from build123d import *

# Parameters (mm, degrees)
F1_DEPTH = 25
F2_R     = 8
F3_DEPTH = 25
F4_SIZE  = 5
F5_R     = 1.75
F6_DEPTH = 25


with BuildPart() as f1:
    # F0 (on Right) → F1 (new body)
    with BuildSketch(Plane.YZ):
        with BuildLine():
            Line((2, 47), (0, 47))
            Line((0, 47), (0, 5))
            ThreePointArc((0, 5), (1.464466, 1.464466), (5, 0))
            Line((5, 0), (52, 0))
            Line((52, 0), (52, 2))
            Line((52, 2), (5, 2))
            ThreePointArc((5, 2), (2.87868, 2.87868), (2, 5))
            Line((2, 5), (2, 47))
        make_face()
    extrude(amount=F1_DEPTH)

    # F2 (on face) → F3 (cut)
    with BuildSketch(Plane(origin=(0, 2, 0), x_dir=(-1, 0, 0), z_dir=(0, 1, 0))):
        with Locations((-12.5, 35)):
            Circle(F2_R)
    extrude(amount=-F3_DEPTH, mode=Mode.SUBTRACT)

    # F4
    f4_edges = [f1.edges().sort_by_distance(p)[0] for p in [
        (0, 1, 47),
        (25, 1, 47),
    ]]
    chamfer(f4_edges, length=F4_SIZE)

    # F5 (on face) → F6 (cut)
    with BuildSketch(Plane.XY.offset(2)):
        with Locations((12.5, 43)):
            Circle(F5_R)
        with Locations((12.5, 28)):
            Circle(F5_R)
    extrude(amount=-F6_DEPTH, mode=Mode.SUBTRACT)


solid = f1.part
CAD build for the part. Positions are in the model's coordinates, mm. A direction names the side the tool comes from. Round coordinates to 2 decimals unless told otherwise and drop trailing zeros. Write each loop counter-clockwise with the first axis right and the second up, starting at its lowest first coordinate (ties: lowest second). Pieces come first, ordered by that corner, then holes. Notation, with made-up numbers: M -17.75,74 L 20.25,74 A35 ccw 20.25,108 Z; hole C -18,8 d8. An arc over 180 degrees is marked long. Use a Markdown table: item, result. Add a question column.
1. Flat gauge pins, fed straight in: P1, Ø5, axis at x = 21.5, y = 26.5, coming from the +Z side; P2, Ø12.5, axis at x = 15.5, z = 24.5, coming from the +Y side. Where does each tip first touch, or does it go through?
2. Slice it at C-C on z = 36. Give the cut face in (x, y).
3. Drill centre lines: probe 1 along Y at (x, z) = (12.5, 1.35); probe 2 along Y at (x, z) = (12.5, 1.5); probe 3 along Z at (x, y) = (8.5, 47). Where is each one in solid material? Low to high.
4. Slice it at A-A on y = 43. Give the cut face in (x, z).
5. Slice it at B-B on x = 12.5. Give the cut face in (y, z), then the cut area to 3 significant figures.
6. 3-axis set-ups, long thin cutter, end or side, ignore diameter. For faces 1 (the face through (12, 2, 21)), 2 (the face through (13.541, 1.014, 42.932)): which of +Z, -Z, +X, -X, +Y, -Y reach the whole face in a straight line?
7. Slice it at D-D on x = 5.75. Give the cut face in (y, z), then the cut area to 3 significant figures.
8. Pull direction X, two halves, no side cores. Call faces 3 (the face through (12, 52, 1)), 4 (the face through (12.12, 41.29, 1.01)), 5 (the face through (14.169, 28.526, 1.014)), 6 (the face through (25, 14, 1)): released by +X, released by -X, zero draft, split by the parting line, or undercut.
Reply:
| question | item | result |
|---|---|---|
| 1 | P1 | stops at z = 2 |
| 1 | P2 | stops at y = 2 |
| 2 | outline | M 0,0 L 4.56,0 L 4.56,2 L 0,2 Z; M 20.44,0 L 25,0 L 25,2 L 20.44,2 Z |
| 3 | probe 1 | y = 1.58 to 26.25, 29.75 to 41.25, 44.75 to 52 |
| 3 | probe 2 | y = 1.43 to 26.25, 29.75 to 41.25, 44.75 to 52 |
| 3 | probe 3 | z = 0 to 2 |
| 4 | outline | M 0,0 L 10.75,0 L 10.75,2 L 0,2 Z; M 14.25,0 L 25,0 L 25,2 L 14.25,2 Z |
| 5 | outline | M 0,5 A5 ccw 5,0 L 26.25,0 L 26.25,2 L 5,2 A3 cw 2,5 L 2,27 L 0,27 Z; M 0,43 L 2,43 L 2,47 L 0,47 Z; M 29.75,0 L 41.25,0 L 41.25,2 L 29.75,2 Z; M 44.75,0 L 52,0 L 52,2 L 44.75,2 Z |
| 5 | area | 145 mm^2 |
| 6 | face 1 | +Z, +X, -X, +Y |
| 6 | face 2 | +Y, -Y |
| 7 | outline | M 0,5 A5 ccw 5,0 L 52,0 L 52,2 L 5,2 A3 cw 2,5 L 2,30.71 L 0,30.71 Z; M 0,39.29 L 2,39.29 L 2,47 L 0,47 Z |
| 7 | area | 173 mm^2 |
| 8 | face 3 | zero draft |
| 8 | face 4 | undercut |
| 8 | face 5 | undercut |
| 8 | face 6 | released by +X |
